from build123d import *
from build123d.topology import SkipClean

# Parameters (mm, degrees)
CUT_EXTRUDE1_DEPTH = 58.15
CIRPATTERN1_COUNT  = 5


with BuildPart() as part:
    # Sketch1 → Revolve1 (revolve)
    with BuildSketch(Plane.XY, mode=Mode.PRIVATE) as revolve1_sk:
        Polygon((38.1, 6.35), (38.1, 0), (0, 0), (0, 6.35), (3.175, 6.35), (3.175, 19.05), (4.7625, 19.05), (4.7625, 2.54), (30.1625, 2.54), (30.1625, 6.35), align=None)
    revolve(revolve1_sk.sketch.rotate(Axis((0, 0, 0), (0, 1, 0)), 90), axis=Axis((0, 0, 0), (0, 1, 0)))

    # Sketch2 → Cut-Extrude1 (cut, through all)
    with SkipClean():  # the faces are left unmerged after this step: merging them gives an invalid solid
        with BuildSketch(Plane.XZ):
            with BuildLine():
                Line((0.599134, 30.156549), (0.599134, 9.836549))
                ThreePointArc((0.599134, 9.836549), (3.139134, 5.43714), (8.219134, 5.43714))
                Line((8.219134, 5.43714), (25.81677, 15.59714))
                ThreePointArc((25.81677, 15.59714), (15.08125, 26.121491), (0.599134, 30.156549))
            make_face()
        cut_extrude1 = extrude(amount=-CUT_EXTRUDE1_DEPTH, mode=Mode.SUBTRACT)

    # CirPattern1: Cut-Extrude1 ×5 about axis
    cirpattern1_axis = Axis((0, 0, 0), (0, 1, 0))
    for i in range(1, CIRPATTERN1_COUNT):
        add(cut_extrude1.rotate(cirpattern1_axis, i * 360 / CIRPATTERN1_COUNT), mode=Mode.SUBTRACT)


solid = part.part
Design review of the part built by this model. Coordinates are the model's own, in mm. A direction names the side the tool comes from. Give positions to 0.01 mm unless a question says otherwise; leave off trailing zeros. Order: outer loops, then holes, each group sorted by start corner. A loop starts at its lowest first (then second) coordinate and runs counter-clockwise, first axis right, second up. Notation, with made-up numbers: (29, 84.25) - (70, 84.25) arc R27 cw to (70, 117.25) - close; hole circle Ø6 at (9.25, -20). An arc over 180 degrees is marked (long way). Use CSV: the item, a comma, the result in double quotes. Start each with the question number.
Q1. Draft analysis for pull direction Z (two halves, no side actions). For faces 3 (the face through (37.194, 3.131, 8.259)), 4 (the face through (0.73, 1.252, -6.237)), 5 (the face through (-1, 0, 1)), state which applies: pulls with the +Z half, pulls with the -Z half, needs draft (parallel to the pull), parting line crosses it, or undercut.
Q2. Take a section at B-B (z = -15). State the section outline as (x, y) points, and give its area (3 significant figures).
Q3. For P1, Ø0.8, axis at y = 1.5, z = 19, coming from the +X side; P2, Ø3, axis at y = 15, z = 7, coming from the +X side; P3, Ø1.9, axis at x = 0.5, z = -0.5, coming from the +Y side; P4, Ø12, axis at x = -8, z = -12.5, coming from the +Y side, all flat-tipped, find the tip position at first contact; note any pin that passes through.
Q4. Take a section at C-C (x = 24.5). State the section outline as (y, z) points, and give its area (3 significant figures).
Q5. Take a section at D-D (z = -29). State the section outline as (x, y) points, and give its area (4 significant figures).
Q6. Take a section at A-A (y = 3.5). State the section outline as (x, z) points (1 decimal).
Q7. For line 1 (X direction, y = 3.9, z = 0); line 2 (X direction, y = 1, z = -4); line 3 (X direction, y = 14, z = 0) (1 decimal), list the stretches that pass through material, from the lowest coordinate up.
Q8. Machinability: for faces 1 (the face through (0, 6.35, 0)), 2 (the face through (19.338, 1.252, 5.653)), which of the approach directions +Z, -Z, +X, -X, +Y, -Y give a long, thin tool a straight path to every point of the face, cutting with its end or side? Answer none if there is none.
Calculated:
1,face 3,"parting line crosses it"
1,face 4,"undercut"
1,face 5,"needs draft"
2,outline,"(-35.02, 0) - (-26.17, 0) - (-26.17, 6.35) - (-35.02, 6.35) - close; (-11.64, 0) - (-6.02, 0) - (-6.02, 2.54) - (-11.64, 2.54) - close; (10.16, 0) - (17.55, 0) - (17.55, 2.54) - (10.16, 2.54) - close; (26.17, 0) - (35.02, 0) - (35.02, 6.35) - (26.17, 6.35) - close"
2,area,"146 mm²"
3,P1,"stops at x = 33.25"
3,P2,"passes through"
3,P3,"stops at y = 6.35"
3,P4,"stops at y = 2.54"
4,outline,"(0, -29.18) - (6.35, -29.18) - (6.35, -17.59) - (0, -17.59) - close; (0, 7.33) - (2.54, 7.33) - (2.54, 14.84) - (0, 14.84) - close; (0, 17.59) - (6.35, 17.59) - (6.35, 29.18) - (0, 29.18) - close"
4,area,"166 mm²"
5,outline,"(-24.71, 0) - (-8.29, 0) - (-8.29, 6.35) - (-24.71, 6.35) - close; (8.29, 0) - (24.71, 0) - (24.71, 6.35) - (8.29, 6.35) - close"
5,area,"208.5 mm²"
6,outline,"circle Ø76.2 at (0, 0); circle Ø9.5 at (0, 0); hole circle Ø60.3 at (0, 0)"
7,line 1,"x = -38.1 to -30.16, -4.76 to 4.76, 30.16 to 38.1"
7,line 2,"x = -37.89 to -29.9, -5.33 to 6.3, 29.9 to 37.89"
7,line 3,"x = -4.8 to -3.2, 3.2 to 4.8"
8,face 1,"+Y"
8,face 2,"+Y, -Y"
